Here's how the part is built. I have some questions about the finished solid (model axes, mm). Face numbers are marked on the shaded views. A direction names the side the tool comes from. Give positions to 0.01 mm unless a question says otherwise; leave off trailing zeros. Loops run counter-clockwise (first coordinate to the right, second up) from the corner with the lowest first, then second, coordinate; pieces in that order, holes last.
Q1. Suppose I cut it at B-B (x = 8.75). List the corners of the cut face in (y, z) for me, and give its area (3 significant figures).
Q2. Suppose I cut it at A-A (z = 3.9). List the corners of the cut face in (x, y) for me.
Q3. Suppose I cut it at D-D (y = 1.5). List the corners of the cut face in (x, z) for me, and give its area (3 significant figures).
Q4. I need wall thicknesses on probe 1 along X at (y, z) = (2.5, 4.35); probe 2 along Y at (x, z) = (9, 2); probe 3 along X at (y, z) = (4, 1.65). Which ranges of each line are inside material? Lowest first, please.
Q5. Thinking about a two-plate mould opening in X: for the marked faces 1, 2 and 3, which applies, pulls with the +X half, pulls with the -X half, needs draft (parallel to the pull), parting line crosses it, or undercut?
Q6. For the marked faces 4 and 5, which set-ups out of +Z, -Z, +X, -X, +Y, -Y let a thin tool reach every point of the face, with its end or its side?
Q7. Suppose I cut it at C-C (y = 2.37). List the corners of the cut face in (x, z) for me, and give its area (4 significant figures).
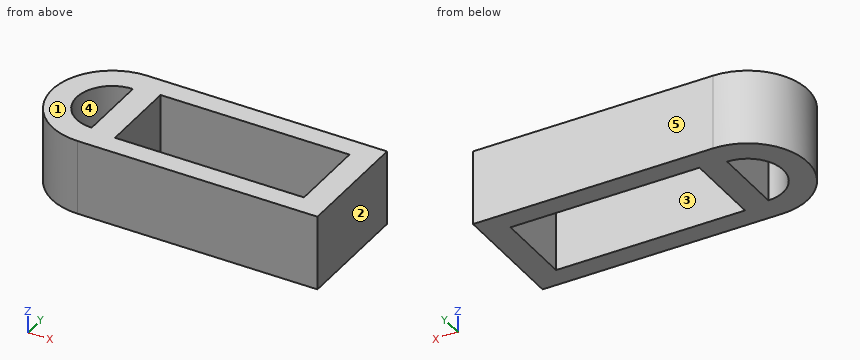
```python
from build123d import *

# Parameters (mm, degrees)
F0_W     = 12.6
F0_H     = 5.24
F1_DEPTH = 5


with BuildPart() as f1:
    # F0 (on Top) → F1 (new body)
    with BuildSketch(Plane.XY):
        with Locations((6.15, 2.37)):
            Rectangle(F0_W, F0_H)
        with BuildLine():
            ThreePointArc((-1.85, 6.37), (-5.85, 2.37), (-1.85, -1.63))
            Line((-1.85, -1.63), (14.15, -1.63))
            Line((14.15, -1.63), (14.15, 6.37))
            Line((14.15, 6.37), (-1.85, 6.37))
        make_face()
        with BuildLine():
            Line((-1.85, 4.74), (-1.85, 0))
            ThreePointArc((-1.85, 0), (-4.22, 2.37), (-1.85, 4.74))
        make_face(mode=Mode.SUBTRACT)
        with Locations((6.15, 2.37)):
            Rectangle(F0_W, F0_H, mode=Mode.SUBTRACT)
    extrude(amount=F1_DEPTH)


solid = f1.part
```
Solutions:
1. outline: (-1.63, 0) - (-0.25, 0) - (-0.25, 5) - (-1.63, 5) - close; (4.99, 0) - (6.37, 0) - (6.37, 5) - (4.99, 5) - close
1. area: 13.8 mm2
2. outline: (-1.85, -1.63) - (14.15, -1.63) - (14.15, 6.37) - (-1.85, 6.37) arc R4 ccw to start; hole (-1.85, 0) - (-1.85, 4.74) arc R2.37 ccw to start; hole (-0.15, -0.25) - (12.45, -0.25) - (12.45, 4.99) - (-0.15, 4.99) - close
3. outline: (-5.75, 0) - (-4.05, 0) - (-4.05, 5) - (-5.75, 5) - close; (-1.85, 0) - (-0.15, 0) - (-0.15, 5) - (-1.85, 5) - close; (12.45, 0) - (14.15, 0) - (14.15, 5) - (12.45, 5) - close
3. area: 25.5 mm2
4. probe 1: x = -5.85 to -4.22, -1.85 to -0.15, 12.45 to 14.15
4. probe 2: y = -1.63 to -0.25, 4.99 to 6.37
4. probe 3: x = -5.5 to -3.57, -1.85 to -0.15, 12.45 to 14.15
5. face 1: needs draft
5. face 2: pulls with the +X half
5. face 3: undercut
6. face 4: +Z, -Z
6. face 5: +Z, -Z, +X, -X, +Y
7. outline: (-5.85, 0) - (-4.22, 0) - (-4.22, 5) - (-5.85, 5) - close; (-1.85, 0) - (-0.15, 0) - (-0.15, 5) - (-1.85, 5) - close; (12.45, 0) - (14.15, 0) - (14.15, 5) - (12.45, 5) - close
7. area: 25.15 mm2
